from build123d import *

# Parameters (mm, degrees)
SKETCH1_W           = 100
SKETCH1_H           = 100
BOSS_EXTRUDE1_DEPTH = 100
CUT_EXTRUDE1_DEPTH  = 100
SKETCH3_R           = 12
CUT_EXTRUDE2_DEPTH  = 80
SKETCH5_R           = 5
CUT_EXTRUDE3_DEPTH  = 50
BOSS_EXTRUDE2_DEPTH = 30
SKETCH8_R           = 10
CUT_EXTRUDE4_DEPTH  = 30
CUT_EXTRUDE5_DEPTH  = 10
SKETCH10_R          = 30
CUT_EXTRUDE6_DEPTH  = 96
CUT_EXTRUDE7_DEPTH  = 30
BOSS_EXTRUDE5_DEPTH = 10
SKETCH15_R          = 30
SKETCH15_R_2        = 12
BOSS_EXTRUDE6_DEPTH = 40
SKETCH16_R          = 12
BOSS_EXTRUDE7_DEPTH = 10
CUT_EXTRUDE8_DEPTH  = 10
CUT_EXTRUDE9_DEPTH  = 20


with BuildPart() as part:
    # Sketch1 → Boss-Extrude1 (new body)
    with BuildSketch(Plane.XY):
        with Locations((50, 50)):
            Rectangle(SKETCH1_W, SKETCH1_H)
    extrude(amount=BOSS_EXTRUDE1_DEPTH)

    # Sketch2 → Cut-Extrude1 (cut)
    with BuildSketch(Plane.XY.offset(100)):
        with BuildLine():
            Line((0, 80), (0, 100))
            Line((0, 100), (20, 100))
            ThreePointArc((20, 100), (5.857864376, 94.142135624), (0, 80))
        make_face()
        with BuildLine():
            Line((80, 100), (100, 100))
            Line((100, 100), (100, 80))
            ThreePointArc((100, 80), (94.142135624, 94.142135624), (80, 100))
        make_face()
        with BuildLine():
            Line((80, 0), (100, 0))
            Line((100, 0), (100, 20))
            ThreePointArc((100, 20), (94.142135624, 5.857864376), (80, 0))
        make_face()
        with BuildLine():
            Line((0, 20), (0, 0))
            Line((0, 0), (20, 0))
            ThreePointArc((20, 0), (5.857864376, 5.857864376), (0, 20))
        make_face()
    extrude(amount=-CUT_EXTRUDE1_DEPTH, mode=Mode.SUBTRACT)

    # Sketch3 → Cut-Extrude2 (cut)
    with BuildSketch(Plane(origin=(0, 0, 0), x_dir=(-1, 0, 0), z_dir=(0, 0, -1))):
        with Locations((-60, 50)):
            Circle(SKETCH3_R)
    extrude(amount=-CUT_EXTRUDE2_DEPTH, mode=Mode.SUBTRACT)

    # Sketch5 → Cut-Extrude3 (cut)
    with BuildSketch(Plane.XY.offset(20)):
        with Locations((20, 50)):
            Circle(SKETCH5_R)
    extrude(amount=CUT_EXTRUDE3_DEPTH, mode=Mode.SUBTRACT)

    # Sketch7 → Boss-Extrude2 (add)
    with BuildSketch(Plane.XY.offset(30)):
        with BuildLine():
            Line((0, 80), (-20, 80))
            ThreePointArc((-20, 80), (-50, 50), (-20, 20))
            Line((-20, 20), (0, 20))
            Line((0, 20), (0, 80))
        make_face()
    extrude(amount=BOSS_EXTRUDE2_DEPTH)

    # Sketch8 → Cut-Extrude4 (cut)
    with BuildSketch(Plane.XY.offset(60)):
        with Locations((-20, 50)):
            Circle(SKETCH8_R)
    extrude(amount=-CUT_EXTRUDE4_DEPTH, mode=Mode.SUBTRACT)

    # Sketch9 → Cut-Extrude5 (cut)
    with BuildSketch(Plane.XY.offset(60)):
        with BuildLine():
            Line((-20, 60), (-48.284271247, 60))
            ThreePointArc((-48.284271247, 60), (-50, 50), (-48.284271247, 40))
            Line((-48.284271247, 40), (-20, 40))
            ThreePointArc((-20, 40), (-30, 50), (-20, 60))
        make_face()
    extrude(amount=-CUT_EXTRUDE5_DEPTH, mode=Mode.SUBTRACT)

    # Sketch10 → Cut-Extrude6 (cut)
    with BuildSketch(Plane.XY.offset(30)):
        with Locations(Location((60, 50, 0), (0, 0, 180))):
            Circle(SKETCH10_R)
    extrude(amount=CUT_EXTRUDE6_DEPTH, mode=Mode.SUBTRACT)

    # Sketch11 → Cut-Extrude7 (cut)
    with BuildSketch(Plane.XY.offset(100)):
        with BuildLine():
            Line((20, 70), (0, 70))
            Line((0, 70), (0, 30))
            Line((0, 30), (20, 30))
            ThreePointArc((20, 30), (40, 50), (20, 70))
        make_face()
    extrude(amount=-CUT_EXTRUDE7_DEPTH, mode=Mode.SUBTRACT)

    # Sketch14 → Boss-Extrude5 (add)
    with BuildSketch(Plane.XY.offset(70)):
        with BuildLine():
            Line((20, 55), (20, 70))
            ThreePointArc((20, 70), (40, 50), (20, 30))
            Line((20, 30), (20, 45))
            ThreePointArc((20, 45), (25, 50), (20, 55))
        make_face()
    extrude(amount=BOSS_EXTRUDE5_DEPTH)

    # Sketch15 → Boss-Extrude6 (add)
    with BuildSketch(Plane.XY.offset(30)):
        with Locations((60, 50)):
            Circle(SKETCH15_R)
        with Locations(Location((60, 50, 0), (0, 0, 180))):
            Circle(SKETCH15_R_2, mode=Mode.SUBTRACT)
    extrude(amount=BOSS_EXTRUDE6_DEPTH)

    # Sketch16 → Boss-Extrude7 (add)
    with BuildSketch(Plane.XY.offset(70)):
        with BuildLine():
            ThreePointArc((33.75, 35.476312452), (90, 50), (33.75, 64.523687548))
            ThreePointArc((33.75, 64.523687548), (40, 50), (33.75, 35.476312452))
        make_face()
        with Locations(Location((60, 50, 0), (0, 0, 180))):
            Circle(SKETCH16_R, mode=Mode.SUBTRACT)
    extrude(amount=BOSS_EXTRUDE7_DEPTH)

    # Sketch17 → Cut-Extrude8 (cut)
    with BuildSketch(Plane.XY.offset(80)):
        with BuildLine():
            Line((20, 70), (20, 55))
            ThreePointArc((20, 55), (25, 50), (20, 45))
            Line((20, 45), (20, 30))
            ThreePointArc((20, 30), (27.400211113, 31.419448999), (33.75, 35.476312452))
            ThreePointArc((33.75, 35.476312452), (40, 50), (33.75, 64.523687548))
            ThreePointArc((33.75, 64.523687548), (27.400211113, 68.580551001), (20, 70))
        make_face()
    extrude(amount=-CUT_EXTRUDE8_DEPTH, mode=Mode.SUBTRACT)

    # Sketch18 → Cut-Extrude9 (cut)
    with BuildSketch(Plane(origin=(0, 0, 0), x_dir=(-1, 0, 0), z_dir=(0, 0, -1))):
        with BuildLine():
            Line((0, 70), (-20, 70))
            ThreePointArc((-20, 70), (-40, 50), (-20, 30))
            Line((-20, 30), (0, 30))
            Line((0, 30), (0, 70))
        make_face()
    extrude(amount=-CUT_EXTRUDE9_DEPTH, mode=Mode.SUBTRACT)


solid = part.part
Design review of the part built by this model. Coordinates are the model's own, in mm. A direction names the side the tool comes from. Coordinates: 2 decimals unless noted, no trailing zeros. Order: outer loops, then holes, each group sorted by start corner. A loop starts at its lowest first (then second) coordinate and runs counter-clockwise, first axis right, second up. Notation, with made-up numbers: M 4,-13.75 L 24,-13.75 A16 cw 24,0.25 Z; hole C -15,30 d3. An arc over 180 degrees is marked long. Use a Markdown table: item, result.
(1) Add section B-B (x = 60). Give the boundary of the cut face in (y, z), then the cut area to 3 significant figures.
Worked answers:
| item | result |
|---|---|
| outline | M 0,0 L 38,0 L 38,80 L 20,80 L 20,100 L 0,100 Z; M 62,0 L 100,0 L 100,100 L 80,100 L 80,80 L 62,80 Z |
| area | 6,880 mm2 |
(2) For faces 5 (the flat face through (10, 70, 10)), 6 (the flat face through (15, 46, 70)), 7 (the flat face through (-31, 50, 30)), 8 (the flat face through (-8, 50, 60)), list the 3-axis set-ups (+Z, -Z, +X, -X, +Y, -Y) from which the entire face can be reached by the end or side of a thin tool; tool diameter is ignored.
Worked answers:
| item | result |
|---|---|
| face 5 | -Z, -X |
| face 6 | +Z, -X |
| face 7 | -Z, -X, +Y, -Y |
| face 8 | +Z, -X, +Y, -Y |
(3) Draft analysis for pull direction X (two halves, no side actions). For faces 1 (the cylindrical face through (-49.993, 50.66, 44.79)), 2 (the cylindrical face through (94.297, 93.986, 50.7)), 3 (the flat face through (74, 50, 80)), 4 (the flat face through (10, 30, 10)), state which applies: released by +X, released by -X, zero draft, split by the parting line, or undercut.
Worked answers:
| item | result |
|---|---|
| face 1 | released by -X |
| face 2 | released by +X |
| face 3 | undercut |
| face 4 | zero draft |
(4) For P1, Ø14.5, axis at x = -26.5, y = 63, coming from the +Z side; P2, Ø2, axis at x = 11, z = 36.5, coming from the -Y side; P3, Ø16, axis at x = -10.5, z = 47, coming from the +Y side; P4, Ø9, axis at x = 20, y = 50, coming from the -Z side, all flat-tipped, find the tip position at first contact; note any pin that passes through.
Worked answers:
| item | result |
|---|---|
| P1 | stops at z = 60 |
| P2 | stops at y = 1.67 |
| P3 | stops at y = 80 |
| P4 | passes through |
(5) Add section C-C (z = 14). Give the boundary of the cut face in (x, y), then the cut area to 3 significant figures.
Worked answers:
| item | result |
|---|---|
| outline | M 0,20 A20 ccw 20,0 L 80,0 A20 ccw 100,20 L 100,80 A20 ccw 80,100 L 20,100 A20 ccw 0,80 L 0,70 L 20,70 A20 cw 20,30 L 0,30 Z; hole C 60,50 d24 |
| area | 7,780 mm2 |
(6) Wall thickness on probe 1 along X at (y, z) = (50, 33); probe 2 along X at (y, z) = (50, 52.5); probe 3 along Y at (x, z) = (20, 38.5): over which ranges is each line inside the solid? List them lowest first.
Worked answers:
| item | result |
|---|---|
| probe 1 | x = -50 to -30, -10 to 15, 25 to 48, 72 to 100 |
| probe 2 | x = -10 to 15, 25 to 48, 72 to 100 |
| probe 3 | y = 0 to 45, 55 to 100 |
(7) Add section D-D (z = 88). Give the boundary of the cut face in (x, y).
Worked answers:
| item | result |
|---|---|
| outline | M 0,20 A20 ccw 20,0 L 80,0 A20 ccw 100,20 L 100,80 A20 ccw 80,100 L 20,100 A20 ccw 0,80 L 0,70 L 20,70 A20 cw 33.75,64.52 A30 cw long 33.75,35.48 A20 cw 20,30 L 0,30 Z |
(8) Add section A-A (y = 50). Give the boundary of the cut face in (x, z), then the cut area to 3 significant figures.
Worked answers:
| item | result |
|---|---|
| outline | M -50,30 L -30,30 L -30,50 L -50,50 Z; M -10,30 L 0,30 L 0,20 L 15,20 L 15,70 L 0,70 L 0,60 L -10,60 Z; M 25,20 L 40,20 L 40,0 L 48,0 L 48,80 L 40,80 L 40,70 L 25,70 Z; M 72,0 L 100,0 L 100,100 L 90,100 L 90,80 L 72,80 Z |
| area | 5,280 mm2 |
